Could you check a few things on this model? Use its own coordinates, in mm. A direction names the side the tool comes from. Coordinates: 2 decimals unless noted, no trailing zeros. Loops run counter-clockwise (first coordinate to the right, second up) from the corner with the lowest first, then second, coordinate; pieces in that order, holes last.
1) Thinking about a two-plate mould opening in Y: for faces 6 (the face through (32.5, 22, -39)), 7 (the face through (52, 6, -39)), 8 (the face through (52, 16, -39)), 9 (the face through (158, 18, -39)), which applies, released by +Y, released by -Y, zero draft, split by the parting line, or undercut?
2) If I drill on line 1 along X through (y, z) = (23.5, -59); line 2 along X through (y, z) = (14, -5); line 3 along Z through (x, y) = (166.5, 16.8), over which ranges is the centre line in solid material (lowest first)?
3) Imagine slicing it at B-B on x = 66. Please give me the cut outline in (y, z), plus the area to 3 significant figures.
4) Will this pin go through, and if not, where does the flat tip stop? P1, Ø12, axis at x = 59.5, z = -49, coming from the +Y side.
5) For faces 1 (the face through (105, 13, -50)), 2 (the face through (210, 13, -40)), 3 (the face through (194, 26, -41)), 4 (the face through (137.5, 11, -39)), 5 (the face through (72.5, 22, -39)), which set-ups out of +Z, -Z, +X, -X, +Y, -Y let a thin tool reach every point of the face, with its end or its side?
6) Imagine slicing it at A-A on y = 8.25. Please give me the cut outline in (x, z), plus the area to 3 significant figures.
7) Imagine slicing it at C-C on z = -66.5. Please give me the cut outline in (x, y), plus the area to 3 significant figures.
```python
from build123d import *

# Parameters (mm, degrees)
BOSS_EXTRUDE1_DEPTH     = 26
SKETCH2_W               = 40
SKETCH2_H               = 20
CUT_EXTRUDE1_DEPTH      = 227.221130755
F_1_4_20_TAPPED_HOLE1_D = 5.1054
SKETCH4_W               = 20
SKETCH4_H               = 20
CUT_EXTRUDE2_DEPTH      = 227.221130755
BOSS_EXTRUDE2_DEPTH     = 80
SKETCH6_R               = 1.3
SKETCH6_W               = 10
SKETCH6_H               = 5
CUT_EXTRUDE3_DEPTH      = 10


with BuildPart() as part:
    # Sketch1 → Boss-Extrude1 (new body)
    with BuildSketch(Plane(origin=(0, 0, 0), x_dir=(1, 0, 0), z_dir=(0, 1, 0))):
        with BuildLine():
            Line((5, 0), (205, 0))
            ThreePointArc((205, 0), (208.535533906, 1.464466094), (210, 5))
            Line((210, 5), (210, 75))
            ThreePointArc((210, 75), (208.535533906, 78.535533906), (205, 80))
            Line((205, 80), (5, 80))
            ThreePointArc((5, 80), (1.464466094, 78.535533906), (0, 75))
            Line((0, 75), (0, 5))
            ThreePointArc((0, 5), (1.464466094, 1.464466094), (5, 0))
        make_face()
    extrude(amount=BOSS_EXTRUDE1_DEPTH)

    # Sketch2 → Cut-Extrude1 (cut, through all)
    with BuildSketch(Plane.XY):
        with Locations((52.5, 16)):
            Rectangle(SKETCH2_W, SKETCH2_H)
        with Locations((157.5, 16)):
            Rectangle(SKETCH2_W, SKETCH2_H)
    extrude(amount=-CUT_EXTRUDE1_DEPTH, mode=Mode.SUBTRACT)

    # 1/4-20 Tapped Hole1 (through all)
    with Locations(Plane(origin=(5, 26, -75), x_dir=(0, 0, 1), z_dir=(0, 1, 0))):
        with Locations((0, 0), (70, 0), (70, 200), (0, 200)):
            Hole(F_1_4_20_TAPPED_HOLE1_D / 2)

    # Sketch4 → Cut-Extrude2 (cut, through all)
    with BuildSketch(Plane(origin=(0, 26, 0), x_dir=(1, 0, 0), z_dir=(0, 1, 0))):
        with Locations((105, 40)):
            Rectangle(SKETCH4_W, SKETCH4_H)
    extrude(amount=-CUT_EXTRUDE2_DEPTH, mode=Mode.SUBTRACT)

    # Sketch5 → Boss-Extrude2 (add)
    with BuildSketch(Plane.XY):
        Polygon((32.5, 18), (27.5, 18), (27.5, 13), (29.5, 13), (29.5, 16), (32.5, 16), (72.5, 16), (75.5, 16), (75.5, 13), (77.5, 13), (77.5, 18), (72.5, 18), align=None)
        Polygon((134.5, 13), (134.5, 16), (137.5, 16), (177.5, 16), (180.5, 16), (180.5, 13), (182.5, 13), (182.5, 18), (177.5, 18), (137.5, 18), (132.5, 18), (132.5, 13), align=None)
    extrude(amount=-BOSS_EXTRUDE2_DEPTH)

    # Sketch6 → Cut-Extrude3 (cut)
    with BuildSketch(Plane(origin=(0, 18, 0), x_dir=(1, 0, 0), z_dir=(0, 1, 0))):
        with Locations(Location((43.5, 45.5, 0), (0, 0, 270))):
            Circle(SKETCH6_R)
        with Locations(Location((43.5, 34.5, 0), (0, 0, 90))):
            Circle(SKETCH6_R)
        with Locations(Location((61.5, 34.5, 0), (0, 0, 270))):
            Circle(SKETCH6_R)
        with Locations(Location((61.5, 45.5, 0), (0, 0, 90))):
            Circle(SKETCH6_R)
        with Locations(Location((148.5, 34.5, 0), (0, 0, 90))):
            Circle(SKETCH6_R)
        with Locations(Location((148.5, 45.5, 0), (0, 0, 270))):
            Circle(SKETCH6_R)
        with Locations(Location((166.5, 45.5, 0), (0, 0, 90))):
            Circle(SKETCH6_R)
        with Locations(Location((166.5, 34.5, 0), (0, 0, 270))):
            Circle(SKETCH6_R)
        with Locations((157.5, 57)):
            Rectangle(SKETCH6_W, SKETCH6_H)
        with Locations((52.5, 57)):
            Rectangle(SKETCH6_W, SKETCH6_H)
    extrude(amount=-CUT_EXTRUDE3_DEPTH, mode=Mode.SUBTRACT)


solid = part.part
```
Filled in:
1. face 6: zero draft
1. face 7: undercut
1. face 8: undercut
1. face 9: released by +Y
2. line 1: x = 0 to 32.5, 72.5 to 137.5, 177.5 to 210
2. line 2: x = 0 to 2.45, 7.55 to 32.5, 72.5 to 137.5, 177.5 to 202.45, 207.55 to 210
2. line 3: z = -80 to -46.8, -44.2 to -35.8, -33.2 to 0
3. outline: (0, -80) - (6, -80) - (6, 0) - (0, 0) - close; (16, -80) - (18, -80) - (18, 0) - (16, 0) - close
3. area: 640 mm2
4. P1: stops at y = 18
5. face 1: +Y, -Y
5. face 2: +Z, -Z, +X, +Y, -Y
5. face 3: +Z, -Z, +X, -X, +Y
5. face 4: +Z, -Z
5. face 5: +Z, -Z, +Y
6. outline: (0, -75) arc R5 ccw to (5, -80) - (32.5, -80) - (32.5, 0) - (5, 0) arc R5 ccw to (0, -5) - close; (72.5, -80) - (137.5, -80) - (137.5, 0) - (72.5, 0) - close; (177.5, -80) - (205, -80) arc R5 ccw to (210, -75) - (210, -5) arc R5 ccw to (205, 0) - (177.5, 0) - close; hole circle Ø5.11 at (5, -75); hole circle Ø5.11 at (5, -5); hole (95, -50) - (115, -50) - (115, -30) - (95, -30) - close; hole circle Ø5.11 at (205, -75); hole circle Ø5.11 at (205, -5)
6. area: 9,900 mm2
7. outline: (0, 0) - (210, 0) - (210, 26) - (177.5, 26) - (177.5, 18) - (137.5, 18) - (137.5, 26) - (72.5, 26) - (72.5, 18) - (32.5, 18) - (32.5, 26) - (0, 26) - close; hole (32.5, 6) - (72.5, 6) - (72.5, 16) - (32.5, 16) - close; hole (137.5, 6) - (177.5, 6) - (177.5, 16) - (137.5, 16) - close
7. area: 4,020 mm2
